Input: dimensioned drawing with shaded views. Units: mm. Origin: part minimum x, y, z. A direction names the side the tool comes from. Coordinates: 2 decimals unless noted, no trailing zeros. Order: outer loops, then holes, each group sorted by start corner. A loop starts at its lowest first (then second) coordinate and runs counter-clockwise, first axis right, second up. Notation, with made-up numbers: (71, 65) -> (104, 65) arc R14 ccw to (104, 83) -> close; hole circle Ø3 at (84.25, 73.5). An arc over 180 degrees is marked (long way). Write item = value, one per line. Start each with the question number.
Item 1: Section query A-A (z = 3.25). Output: boundary loops of the cut face in (x, y).
Item 2: Section query B-B (x = 5.5). Output: boundary loops of the cut face in (y, z).
Item 3: Contact query for a flat-ended pin moving along its axis: pin 1 (1.4 mm diameter, centred on x = 4, y = 1.5, fed in from +Z). Output: stop coordinate, or through.
Item 4: Section query C-C (y = 1.3). Output: boundary loops of the cut face in (x, z).
Item 5: Set-up query: the marked faces 5, 6 and 7. Return all of +Z, -Z, +X, -X, +Y, -Y with unobstructed straight access to the full face (end or side cutting, diameter ignored); none if empty.
Item 6: Section query D-D (x = 1.58). Output: boundary loops of the cut face in (y, z).
Item 7: Mould query, pull axis Y, two halves, no side actions, for the marked faces 1, 2, 3 and 4. Classes: released by +Y, released by -Y, zero draft, split by the parting line, or undercut.
Item 8: Ray query, line 1 along Y through (x, z) = (6, 4); line 2 along Y through (x, z) = (7, 5.5) (1 decimal); line 3 along Y through (x, z) = (1.5, 7). Return the intervals inside material, ascending. Write a range as [from, to].
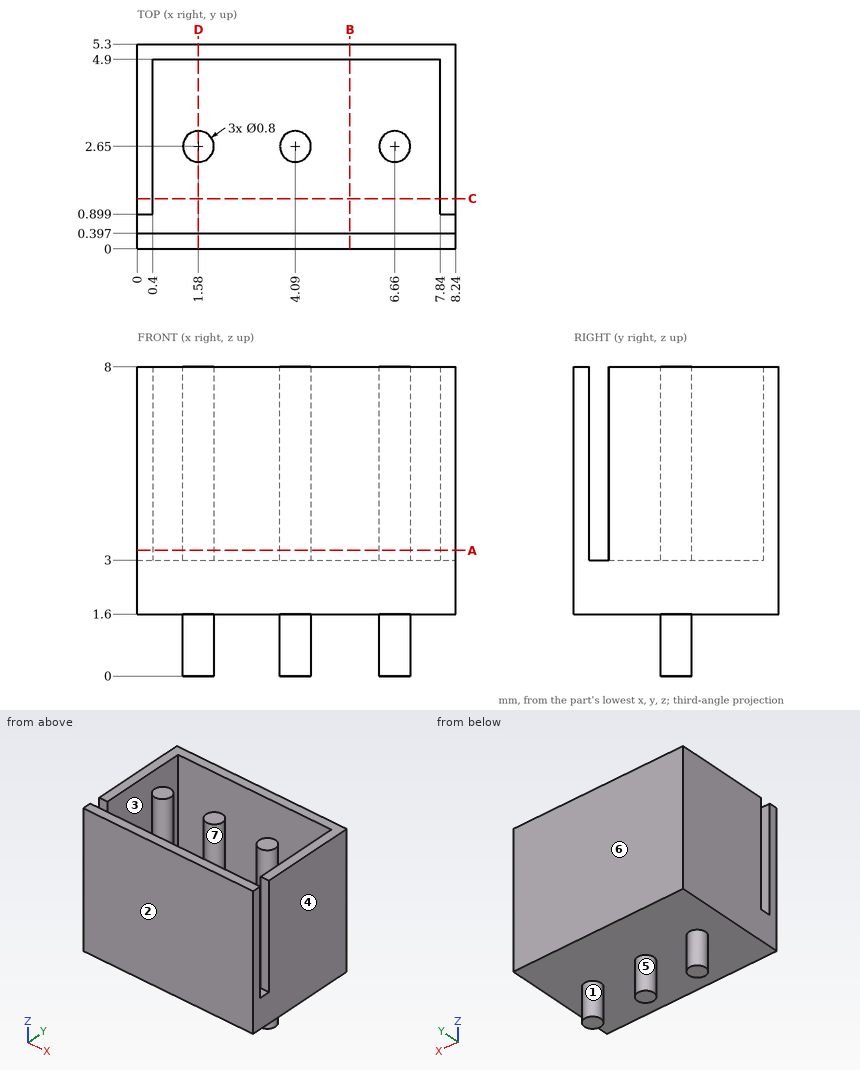
Computed:
q1.outline = (0, 0) -> (8.24, 0) -> (8.24, 0.4) -> (0, 0.4) -> close; (0, 0.9) -> (0.4, 0.9) -> (0.4, 4.9) -> (7.84, 4.9) -> (7.84, 0.9) -> (8.24, 0.9) -> (8.24, 5.3) -> (0, 5.3) -> close; circle Ø0.8 at (1.58, 2.65); circle Ø0.8 at (4.09, 2.65); circle Ø0.8 at (6.66, 2.65)
q2.outline = (0, 1.6) -> (5.3, 1.6) -> (5.3, 8) -> (4.9, 8) -> (4.9, 3) -> (0.4, 3) -> (0.4, 8) -> (0, 8) -> close
q3.pin_1 = 3
q4.outline = (0, 1.6) -> (8.24, 1.6) -> (8.24, 8) -> (7.84, 8) -> (7.84, 3) -> (0.4, 3) -> (0.4, 8) -> (0, 8) -> close
q5.face_5 = -Z
q5.face_6 = +Z, -Z, +X, -X, +Y
q5.face_7 = +Z
q6.outline = (0, 1.6) -> (2.25, 1.6) -> (2.25, 0) -> (3.05, 0) -> (3.05, 1.6) -> (5.3, 1.6) -> (5.3, 8) -> (4.9, 8) -> (4.9, 3) -> (3.05, 3) -> (3.05, 8) -> (2.25, 8) -> (2.25, 3) -> (0.4, 3) -> (0.4, 8) -> (0, 8) -> close
q7.face_1 = split by the parting line
q7.face_2 = released by -Y
q7.face_3 = undercut
q7.face_4 = zero draft
q8.line_1 = [0, 0.4], [4.9, 5.3]
q8.line_2 = [0, 0.4], [2.4, 2.9], [4.9, 5.3]
q8.line_3 = [0, 0.4], [2.26, 3.04], [4.9, 5.3]
